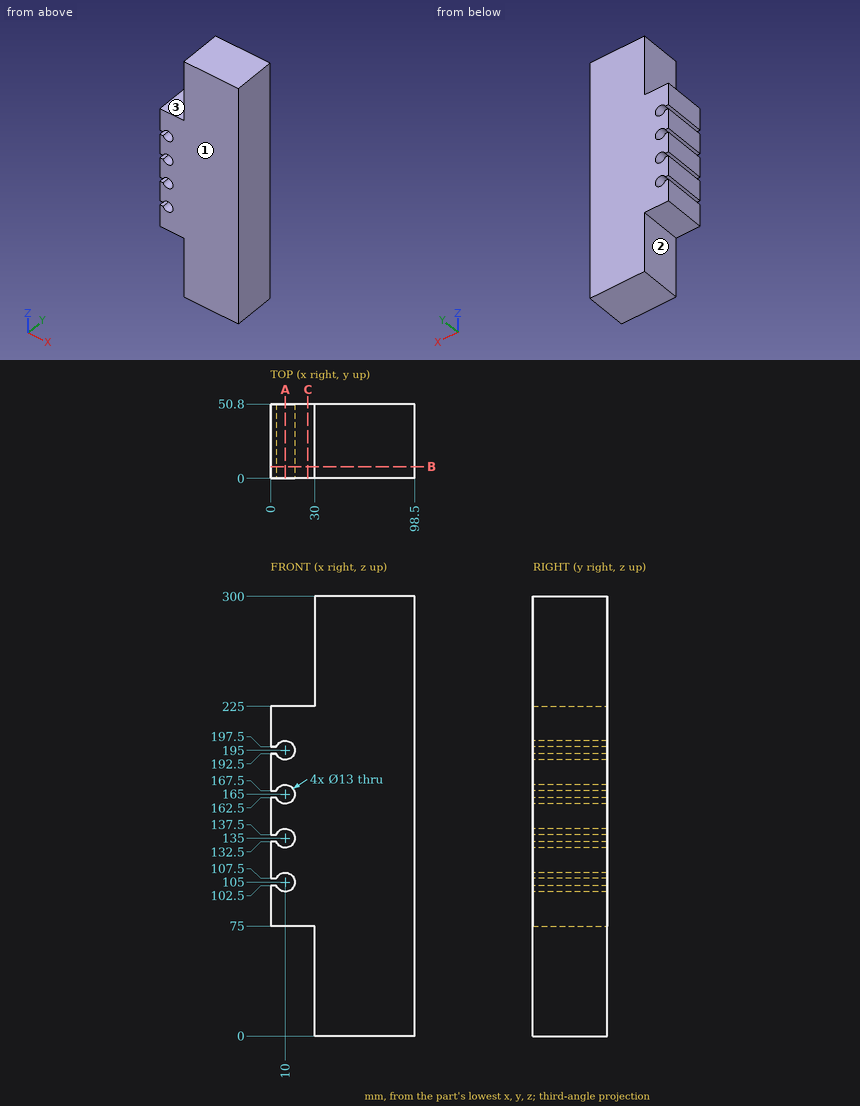
Input: dimensioned drawing with shaded views. Units: mm. Origin: part minimum x, y, z. A direction names the side the tool comes from. Round coordinates to 2 decimals unless told otherwise and drop trailing zeros. Loops run counter-clockwise (first coordinate to the right, second up) from the corner with the lowest first, then second, coordinate; pieces in that order, holes last. Notation, with made-up numbers: M -30,7 L 1,7 A18 ccw 1,18 Z; hole C 71,42 d3. An arc over 180 degrees is marked long. Answer in a Markdown table with one row per item. Add a question column.
1. Section C-C (x = 25.5). Output: boundary loops of the cut face in (y, z), and give its area (3 significant figures).
2. Section A-A (x = 10). Output: boundary loops of the cut face in (y, z), and give its area (3 significant figures).
3. Contact query for flat-ended pins moving along their axis: pin 1 (1.2 mm diameter, centred on x = 2.5, y = 16, fed in from -Z); pin 2 (3 mm diameter, centred on x = 1.5, y = 35, fed in from +Z). Output: stop coordinate, or through.
4. Ray query, probe 1 along Z at (x, y) = (10, 16.5); probe 2 along Z at (x, y) = (7.5, 26); probe 3 along Z at (x, y) = (26.5, 23). Return the intervals inside material, ascending.
5. Section B-B (y = 8). Output: boundary loops of the cut face in (x, z).
6. Set-up query: the marked faces 1, 2 and 3. Return all of +Z, -Z, +X, -X, +Y, -Y with unobstructed straight access to the full face (end or side cutting, diameter ignored); none if empty.
Values follow:
| question | item | result |
|---|---|---|
| 1 | outline | M 0,75 L 50.8,75 L 50.8,225 L 0,225 Z |
| 1 | area | 7,620 mm^2 |
| 2 | outline | M 0,75 L 50.8,75 L 50.8,98.5 L 0,98.5 Z; M 0,111.5 L 50.8,111.5 L 50.8,128.5 L 0,128.5 Z; M 0,141.5 L 50.8,141.5 L 50.8,158.5 L 0,158.5 Z; M 0,171.5 L 50.8,171.5 L 50.8,188.5 L 0,188.5 Z; M 0,201.5 L 50.8,201.5 L 50.8,225 L 0,225 Z |
| 2 | area | 4,980 mm^2 |
| 3 | pin 1 | z = 75 |
| 3 | pin 2 | z = 225 |
| 4 | probe 1 | 75 to 98.5, 111.5 to 128.5, 141.5 to 158.5, 171.5 to 188.5, 201.5 to 225 |
| 4 | probe 2 | 75 to 99, 111 to 129, 141 to 159, 171 to 189, 201 to 225 |
| 4 | probe 3 | 75 to 225 |
| 5 | outline | M 0,75 L 30,75 L 30,0 L 98.5,0 L 98.5,300 L 30,300 L 30,225 L 0,225 L 0,197.5 L 4,197.5 A6.5 cw long 4,192.5 L 0,192.5 L 0,167.5 L 4,167.5 A6.5 cw long 4,162.5 L 0,162.5 L 0,137.5 L 4,137.5 A6.5 cw long 4,132.5 L 0,132.5 L 0,107.5 L 4,107.5 A6.5 cw long 4,102.5 L 0,102.5 Z |
| 6 | face 1 | +Z, -Z, +X, -X, -Y |
| 6 | face 2 | -Z, -X, +Y, -Y |
| 6 | face 3 | +Z, -X, +Y, -Y |
